Design review of the part built by this model. Coordinates are the model's own, in mm. Coordinates: 2 decimals unless noted, no trailing zeros. Loops run counter-clockwise (first coordinate to the right, second up) from the corner with the lowest first, then second, coordinate; pieces in that order, holes last. Notation, with made-up numbers: (-18, 11.5) - (13, 11.5) arc R22 cw to (13, 45.5) - close; hole circle Ø9 at (-33, -21.5). An arc over 180 degrees is marked (long way). Answer in a Markdown table with one row per item. Add a question column.
(1) The part is to be moulded in two halves that separate along X. For faces 1 (the face through (-14.985, -0.56, 0.66)), 2 (the face through (-1, -38, 39)), 3 (the face through (40, 0, 0)), say which applies: released by +X, released by -X, zero draft, split by the parting line, or undercut.
(2) We need section C-C, the plane y = 27. Write out the cut boundary in (x, z), plus the area to 3 significant figures.
(3) Clearance check with a flat-ended pin moving along its axis: pin 1 (6 mm diameter, centred on x = 11.5, z = -6, fed in from -Y). State where the tip first meets the part, or that it passes through.
(4) We need section A-A, the plane x = 0. Write out the cut boundary in (y, z), plus the area to 3 significant figures.
(5) We need section B-B, the plane z = 0. Write out the cut boundary in (x, y), plus the area to 3 significant figures.
(6) To check wall thickness, follow L1, parallel to Z at x = 0, y = -9; L2, parallel to Y at x = 35.5, z = 27; L3, parallel to X at y = 2, z = -8. State the ranges of each line that lie inside material, in increasing order. Write a range as [from, to].
from build123d import *

# Parameters (mm, degrees)
F0_W         = 80
F0_H         = 80
F1_DEPTH     = 40
F2_R         = 5
F3_T1_DEPTH  = 82.5
F3_S5_W      = 5.1
F3_S5_H      = 5.1
F3_T6_DEPTH  = 5.1
F3_S11_W     = 5.1
F3_S11_H     = 5.1
F3_T12_DEPTH = 5.1
F4_R         = 15
F5_DEPTH     = 80.001


# Not quite as in the source:
# - a fillet or chamfer that OpenCascade refuses, or shapes differently, is made with other operations: its cross-section is extruded or revolved along the edge and cut away or added


with BuildPart() as f1:
    # F0 (on Top) → F1 (new body, symmetric)
    with BuildSketch(Plane.XY):
        Rectangle(F0_W, F0_H)
    extrude(amount=F1_DEPTH, both=True)

    # F2
    f2_edges = [f1.edges().sort_by_distance(p)[0] for p in [
        (0, -40, 40),
        (-40, -40, 0),
        (40, -40, 0),
        (0, -40, -40),
        (40, 0, 40),
        (40, 40, 0),
        (40, 0, -40),
        (0, 40, 40),
        (-40, 40, 0),
        (0, 40, -40),
    ]]
    fillet(f2_edges, radius=F2_R)

    # F3: fillet of radius 5 on 6 edges, made by hand

    # F3_s2 → F3_t1 (cut)
    with BuildSketch(Plane.XZ.offset(-35)):
        with BuildLine():
            ThreePointArc((-35, 40), (-38.5355339059, 38.5355339059), (-40, 35))
            Line((-40, 35), (-40, 40))
            Line((-40, 40), (-35, 40))
        make_face()
        with BuildLine():
            ThreePointArc((-35, -40), (-38.5355339059, -38.5355339059), (-40, -35))
            Line((-40, -35), (-40, -40))
            Line((-40, -40), (-35, -40))
        make_face()
    extrude(amount=F3_T1_DEPTH, mode=Mode.SUBTRACT)


with BuildPart() as f3_tool4:
    # F3_s5 → F3_t6 (new body)
    with BuildSketch(Plane.XY.offset(-35)):
        with Locations((-37.55, 37.55)):
            Rectangle(F3_S5_W, F3_S5_H)
    extrude(amount=-F3_T6_DEPTH)

    # F3_s7 → F3_t8 (revolve, cut)
    with BuildSketch(Plane(origin=(-35, 35, -35), x_dir=(0.7071067812, -0.7071067812, 0), z_dir=(0.7071067812, 0.7071067812, 0))):
        with BuildLine():
            ThreePointArc((0, -5), (5, 0), (0, 5))
            Line((0, 5), (0, -5))
        make_face()
    revolve(axis=Axis((-35, 35, -35), (0, 0, -1)), mode=Mode.SUBTRACT)


with BuildPart() as f1_1:
    add(f1.part)

    # F3_t3: cut F3_tool4
    add(f3_tool4.part, mode=Mode.SUBTRACT)


with BuildPart() as f3_tool10:
    # F3_s11 → F3_t12 (new body)
    with BuildSketch(Plane.XY.offset(35)):
        with Locations((-37.55, 37.55)):
            Rectangle(F3_S11_W, F3_S11_H)
    extrude(amount=F3_T12_DEPTH)

    # F3_s13 → F3_t14 (revolve, cut)
    with BuildSketch(Plane(origin=(-35, 35, 35), x_dir=(0.7071067812, -0.7071067812, 0), z_dir=(-0.7071067812, -0.7071067812, 0))):
        with BuildLine():
            ThreePointArc((0, -5), (5, 0), (0, 5))
            Line((0, 5), (0, -5))
        make_face()
    revolve(axis=Axis((-35, 35, 35), (0, 0, 1)), mode=Mode.SUBTRACT)


with BuildPart() as f1_2:
    add(f1_1.part)

    # F3_t9: cut F3_tool10
    add(f3_tool10.part, mode=Mode.SUBTRACT)

    # F4 (on face) → F5 (cut, through all)
    with BuildSketch(Plane.XZ.offset(40)):
        Circle(F4_R)
    extrude(amount=-F5_DEPTH, mode=Mode.SUBTRACT)


solid = f1_2.part
Responses:
| question | item | result |
|---|---|---|
| 1 | face 1 | undercut |
| 1 | face 2 | zero draft |
| 1 | face 3 | released by +X |
| 2 | outline | (-40, -35) arc R5 ccw to (-35, -40) - (35, -40) arc R5 ccw to (40, -35) - (40, 35) arc R5 ccw to (35, 40) - (-35, 40) arc R5 ccw to (-40, 35) - close; hole circle Ø30 at (0, 0) |
| 2 | area | 5,670 mm2 |
| 3 | pin 1 | stops at y = -40 |
| 4 | outline | (-40, -35) arc R5 ccw to (-35, -40) - (35, -40) arc R5 ccw to (40, -35) - (40, -15) - (-40, -15) - close; (-40, 15) - (40, 15) - (40, 35) arc R5 ccw to (35, 40) - (-35, 40) arc R5 ccw to (-40, 35) - close |
| 4 | area | 3,980 mm2 |
| 5 | outline | (-40, -35) arc R5 ccw to (-35, -40) - (-15, -40) - (-15, 40) - (-35, 40) arc R5 ccw to (-40, 35) - close; (15, -40) - (35, -40) arc R5 ccw to (40, -35) - (40, 35) arc R5 ccw to (35, 40) - (15, 40) - close |
| 5 | area | 3,980 mm2 |
| 6 | L1 | z = [-40, -15], [15, 40] |
| 6 | L2 | y = [-39.97, 39.97] |
| 6 | L3 | x = [-40, -12.69], [12.69, 40] |
